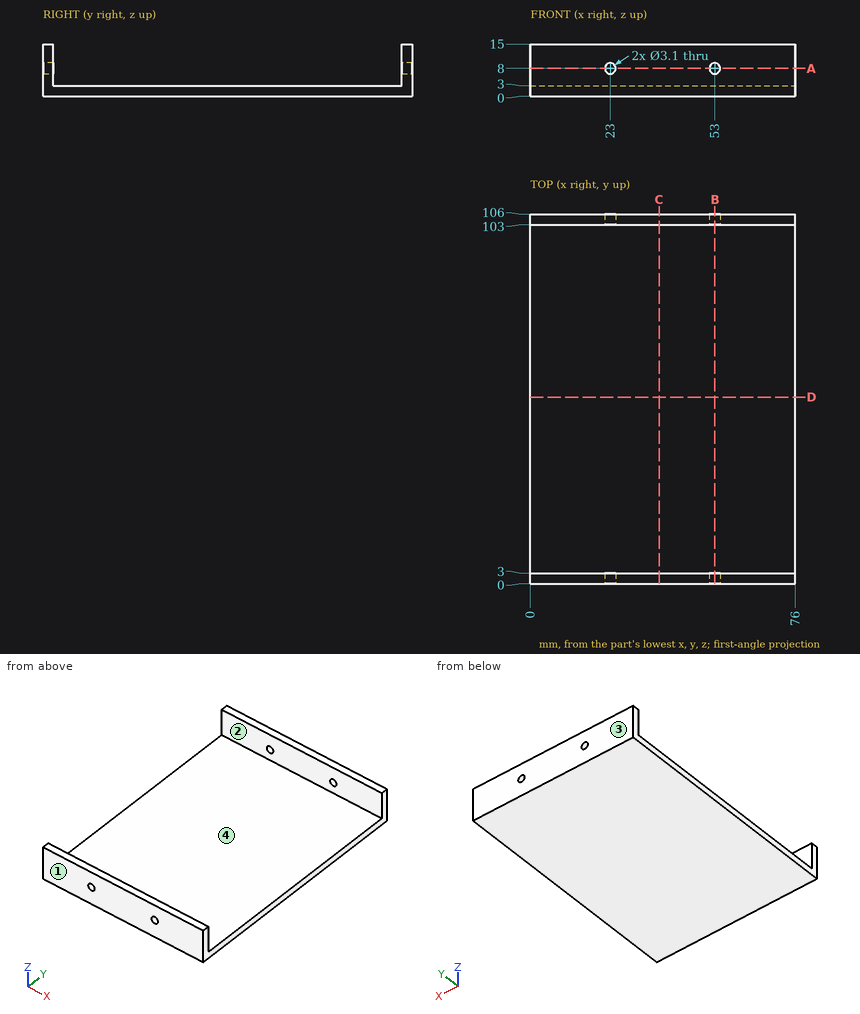
Study the drawing (mm; zero at the part's minimum x, y, z) and answer. Coordinates: 2 decimals unless noted, no trailing zeros. Write each loop counter-clockwise with the first axis right and the second up, starting at its lowest first coordinate (ties: lowest second). Pieces come first, ordered by that corner, then holes. Notation, with made-up numbers: (9.5, 38.5) -> (60.5, 38.5) arc R14 ccw to (60.5, 53.5) -> close; hole circle Ø6 at (-3, 82.25). An arc over 180 degrees is marked (long way). Write each question's results on one line, items separated by ' | '. Start each with the question number.
1) A cutting plane is placed at A-A (z = 8). Determine the outline of the cut face in (x, y), then the cut area to 3 significant figures.
2) A cutting plane is placed at D-D (y = 53.5). Determine the outline of the cut face in (x, z).
3) Straight lines are drawn through the part: probe 1 along X at (y, z) = (1.7, 8); probe 2 along Y at (x, z) = (14.5, 3.75); probe 3 along Z at (x, y) = (4.5, 63). For each, find the intervals that lie inside material, in ascending order.
4) Flat-ended cylindrical pins translate along their axes: pin 1 Ø1.9 at (x, z) = (23, 8) entering from -Y; pin 2 Ø5 at (x, z) = (23, 8) entering from -Y; pin 3 Ø5 at (x, y) = (54.5, 43.5) entering from +Z. Find the tip coordinate at first contact, or state that the pin passes through.
5) For a pull along Y with two mould halves and no side action, classify the marked faces 1, 2, 3 and 4 as +Y half, -Y half, draft (parallel to the pull), parting line (faces both ways), or undercut.
6) A cutting plane is placed at C-C (x = 37). Determine the outline of the cut face in (y, z).
7) A cutting plane is placed at B-B (x = 53). Determine the outline of the cut face in (y, z), then the cut area to 3 significant figures.
Values follow:
1) outline: (0, 0) -> (21.45, 0) -> (21.45, 3) -> (0, 3) -> close; (0, 103) -> (21.45, 103) -> (21.45, 106) -> (0, 106) -> close; (24.55, 0) -> (51.45, 0) -> (51.45, 3) -> (24.55, 3) -> close; (24.55, 103) -> (51.45, 103) -> (51.45, 106) -> (24.55, 106) -> close; (54.55, 0) -> (76, 0) -> (76, 3) -> (54.55, 3) -> close; (54.55, 103) -> (76, 103) -> (76, 106) -> (54.55, 106) -> close | area: 419 mm²
2) outline: (0, 0) -> (76, 0) -> (76, 3) -> (0, 3) -> close
3) probe 1: 0 to 21.45, 24.55 to 51.45, 54.55 to 76 | probe 2: 0 to 3, 103 to 106 | probe 3: 0 to 3
4) pin 1: through | pin 2: y = 0 | pin 3: z = 3
5) face 1: -Y half | face 2: undercut | face 3: +Y half | face 4: undercut
6) outline: (0, 0) -> (106, 0) -> (106, 15) -> (103, 15) -> (103, 3) -> (3, 3) -> (3, 15) -> (0, 15) -> close
7) outline: (0, 0) -> (106, 0) -> (106, 6.45) -> (103, 6.45) -> (103, 3) -> (3, 3) -> (3, 6.45) -> (0, 6.45) -> close; (0, 9.55) -> (3, 9.55) -> (3, 15) -> (0, 15) -> close; (103, 9.55) -> (106, 9.55) -> (106, 15) -> (103, 15) -> close | area: 371 mm²
